```python
from build123d import *

# Parameters (mm, degrees)
F1_DEPTH = 0.15
F2_DEPTH = 1.9
F3_W     = 0.15
F3_H     = 7
F4_DEPTH = 8
F6_DEPTH = 25
F7_R     = 0.5


with BuildPart() as f1:
    # F0 (on Top) → F1 (new body)
    with BuildSketch(Plane.XY):
        with BuildLine():
            Line((96.425, -0.5), (96.425, -3.5))
            Line((96.425, -3.5), (99.425, -3.5))
            Line((99.425, -3.5), (110.2, -3.5))
            Line((110.2, -3.5), (123.975, -3.5))
            Line((123.975, -3.5), (123.975, -0.5))
            Line((123.975, -0.5), (119.375, -0.5))
            ThreePointArc((119.375, -0.5), (119.0921572875, -0.3828427125), (118.975, -0.1))
            Line((118.975, -0.1), (118.975, 0.1))
            ThreePointArc((118.975, 0.1), (119.0921572875, 0.3828427125), (119.375, 0.5))
            Line((119.375, 0.5), (123.975, 0.5))
            Line((123.975, 0.5), (123.975, 3.5))
            Line((123.975, 3.5), (110.2, 3.5))
            Line((110.2, 3.5), (99.425, 3.5))
            Line((99.425, 3.5), (96.425, 3.5))
            Line((96.425, 3.5), (96.425, 0.5))
            Line((96.425, 0.5), (101.025, 0.5))
            ThreePointArc((101.025, 0.5), (101.3078427125, 0.3828427125), (101.425, 0.1))
            Line((101.425, 0.1), (101.425, -0.1))
            ThreePointArc((101.425, -0.1), (101.3078427125, -0.3828427125), (101.025, -0.5))
            Line((101.025, -0.5), (96.425, -0.5))
        make_face()
        with BuildLine():
            Line((13.775, -0.5), (13.775, -3.5))
            Line((13.775, -3.5), (27.55, -3.5))
            Line((27.55, -3.5), (41.325, -3.5))
            Line((41.325, -3.5), (41.325, -0.5))
            Line((41.325, -0.5), (36.725, -0.5))
            ThreePointArc((36.725, -0.5), (36.4421572875, -0.3828427125), (36.325, -0.1))
            Line((36.325, -0.1), (36.325, 0.1))
            ThreePointArc((36.325, 0.1), (36.4421572875, 0.3828427125), (36.725, 0.5))
            Line((36.725, 0.5), (41.325, 0.5))
            Line((41.325, 0.5), (41.325, 3.5))
            Line((41.325, 3.5), (27.55, 3.5))
            Line((27.55, 3.5), (13.775, 3.5))
            Line((13.775, 3.5), (13.775, 0.5))
            Line((13.775, 0.5), (18.375, 0.5))
            ThreePointArc((18.375, 0.5), (18.6578427125, 0.3828427125), (18.775, 0.1))
            Line((18.775, 0.1), (18.775, -0.1))
            ThreePointArc((18.775, -0.1), (18.6578427125, -0.3828427125), (18.375, -0.5))
            Line((18.375, -0.5), (13.775, -0.5))
        make_face()
        with BuildLine():
            Line((41.325, -0.5), (41.325, -3.5))
            Line((41.325, -3.5), (55.1, -3.5))
            Line((55.1, -3.5), (68.875, -3.5))
            Line((68.875, -3.5), (68.875, -0.5))
            Line((68.875, -0.5), (64.275, -0.5))
            ThreePointArc((64.275, -0.5), (63.9921572875, -0.3828427125), (63.875, -0.1))
            Line((63.875, -0.1), (63.875, 0.1))
            ThreePointArc((63.875, 0.1), (63.9921572875, 0.3828427125), (64.275, 0.5))
            Line((64.275, 0.5), (68.875, 0.5))
            Line((68.875, 0.5), (68.875, 3.5))
            Line((68.875, 3.5), (55.1, 3.5))
            Line((55.1, 3.5), (41.325, 3.5))
            Line((41.325, 3.5), (41.325, 0.5))
            Line((41.325, 0.5), (45.925, 0.5))
            ThreePointArc((45.925, 0.5), (46.2078427125, 0.3828427125), (46.325, 0.1))
            Line((46.325, 0.1), (46.325, -0.1))
            ThreePointArc((46.325, -0.1), (46.2078427125, -0.3828427125), (45.925, -0.5))
            Line((45.925, -0.5), (41.325, -0.5))
        make_face()
        with BuildLine():
            Line((68.875, -0.5), (68.875, -3.5))
            Line((68.875, -3.5), (82.65, -3.5))
            Line((82.65, -3.5), (96.425, -3.5))
            Line((96.425, -3.5), (96.425, -0.5))
            Line((96.425, -0.5), (91.825, -0.5))
            ThreePointArc((91.825, -0.5), (91.5421572875, -0.3828427125), (91.425, -0.1))
            Line((91.425, -0.1), (91.425, 0.1))
            ThreePointArc((91.425, 0.1), (91.5421572875, 0.3828427125), (91.825, 0.5))
            Line((91.825, 0.5), (96.425, 0.5))
            Line((96.425, 0.5), (96.425, 3.5))
            Line((96.425, 3.5), (82.65, 3.5))
            Line((82.65, 3.5), (68.875, 3.5))
            Line((68.875, 3.5), (68.875, 0.5))
            Line((68.875, 0.5), (73.475, 0.5))
            ThreePointArc((73.475, 0.5), (73.7578427125, 0.3828427125), (73.875, 0.1))
            Line((73.875, 0.1), (73.875, -0.1))
            ThreePointArc((73.875, -0.1), (73.7578427125, -0.3828427125), (73.475, -0.5))
            Line((73.475, -0.5), (68.875, -0.5))
        make_face()
        with BuildLine():
            Line((0, 3.5), (0, -3.5))
            Line((0, -3.5), (13.775, -3.5))
            Line((13.775, -3.5), (13.775, -0.5))
            Line((13.775, -0.5), (9.175, -0.5))
            ThreePointArc((9.175, -0.5), (8.8921572875, -0.3828427125), (8.775, -0.1))
            Line((8.775, -0.1), (8.775, 0.1))
            ThreePointArc((8.775, 0.1), (8.8921572875, 0.3828427125), (9.175, 0.5))
            Line((9.175, 0.5), (13.775, 0.5))
            Line((13.775, 0.5), (13.775, 3.5))
            Line((13.775, 3.5), (0, 3.5))
        make_face()
        with BuildLine():
            Line((123.975, -0.5), (123.975, -3.5))
            Line((123.975, -3.5), (137.75, -3.5))
            Line((137.75, -3.5), (151.525, -3.5))
            Line((151.525, -3.5), (151.525, -0.5))
            Line((151.525, -0.5), (146.925, -0.5))
            ThreePointArc((146.925, -0.5), (146.6421572875, -0.3828427125), (146.525, -0.1))
            Line((146.525, -0.1), (146.525, 0.1))
            ThreePointArc((146.525, 0.1), (146.6421572875, 0.3828427125), (146.925, 0.5))
            Line((146.925, 0.5), (151.525, 0.5))
            Line((151.525, 0.5), (151.525, 3.5))
            Line((151.525, 3.5), (137.75, 3.5))
            Line((137.75, 3.5), (123.975, 3.5))
            Line((123.975, 3.5), (123.975, 0.5))
            Line((123.975, 0.5), (128.575, 0.5))
            ThreePointArc((128.575, 0.5), (128.8578427125, 0.3828427125), (128.975, 0.1))
            Line((128.975, 0.1), (128.975, -0.1))
            ThreePointArc((128.975, -0.1), (128.8578427125, -0.3828427125), (128.575, -0.5))
            Line((128.575, -0.5), (123.975, -0.5))
        make_face()
        with BuildLine():
            Line((151.525, -0.5), (151.525, -3.5))
            Line((151.525, -3.5), (165.3, -3.5))
            Line((165.3, -3.5), (179.075, -3.5))
            Line((179.075, -3.5), (179.075, -0.5))
            Line((179.075, -0.5), (174.475, -0.5))
            ThreePointArc((174.475, -0.5), (174.1921572875, -0.3828427125), (174.075, -0.1))
            Line((174.075, -0.1), (174.075, 0.1))
            ThreePointArc((174.075, 0.1), (174.1921572875, 0.3828427125), (174.475, 0.5))
            Line((174.475, 0.5), (179.075, 0.5))
            Line((179.075, 0.5), (179.075, 3.5))
            Line((179.075, 3.5), (165.3, 3.5))
            Line((165.3, 3.5), (151.525, 3.5))
            Line((151.525, 3.5), (151.525, 0.5))
            Line((151.525, 0.5), (156.125, 0.5))
            ThreePointArc((156.125, 0.5), (156.4078427125, 0.3828427125), (156.525, 0.1))
            Line((156.525, 0.1), (156.525, -0.1))
            ThreePointArc((156.525, -0.1), (156.4078427125, -0.3828427125), (156.125, -0.5))
            Line((156.125, -0.5), (151.525, -0.5))
        make_face()
        with BuildLine():
            Line((179.075, -0.5), (179.075, -3.5))
            Line((179.075, -3.5), (192.85, -3.5))
            Line((192.85, -3.5), (206.625, -3.5))
            Line((206.625, -3.5), (206.625, -0.5))
            Line((206.625, -0.5), (202.025, -0.5))
            ThreePointArc((202.025, -0.5), (201.7421572875, -0.3828427125), (201.625, -0.1))
            Line((201.625, -0.1), (201.625, 0.1))
            ThreePointArc((201.625, 0.1), (201.7421572875, 0.3828427125), (202.025, 0.5))
            Line((202.025, 0.5), (206.625, 0.5))
            Line((206.625, 0.5), (206.625, 3.5))
            Line((206.625, 3.5), (192.85, 3.5))
            Line((192.85, 3.5), (179.075, 3.5))
            Line((179.075, 3.5), (179.075, 0.5))
            Line((179.075, 0.5), (183.675, 0.5))
            ThreePointArc((183.675, 0.5), (183.9578427125, 0.3828427125), (184.075, 0.1))
            Line((184.075, 0.1), (184.075, -0.1))
            ThreePointArc((184.075, -0.1), (183.9578427125, -0.3828427125), (183.675, -0.5))
            Line((183.675, -0.5), (179.075, -0.5))
        make_face()
    extrude(amount=F1_DEPTH)

    # F2 (add): a face of the model
    f2_faces = [f1.faces().sort_by_distance(p)[0] for p in [
        (0, 0, 0.075),
    ]]
    extrude(f2_faces, amount=F2_DEPTH)

    # F3 (on face) → F4 (join)
    with BuildSketch(Plane(origin=(0, 0, 0), x_dir=(1, 0, 0), z_dir=(0, 0, -1))):
        with Locations((-1.825, 0)):
            Rectangle(F3_W, F3_H)
    extrude(amount=F4_DEPTH)

    # F5 (on face) → F6 (cut)
    with BuildSketch(Plane(origin=(-1.9, 0, 0), x_dir=(0, -1, 0), z_dir=(-1, 0, 0))):
        with BuildLine():
            ThreePointArc((0.5, -7.1), (0.3828427125, -6.8171572875), (0.1, -6.7))
            Line((0.1, -6.7), (-0.1, -6.7))
            ThreePointArc((-0.1, -6.7), (-0.3828427125, -6.8171572875), (-0.5, -7.1))
            Line((-0.5, -7.1), (-0.5, -8))
            Line((-0.5, -8), (0.5, -8))
            Line((0.5, -8), (0.5, -7.1))
        make_face()
    extrude(amount=-F6_DEPTH, mode=Mode.SUBTRACT)

    # F7
    f7_edges = [f1.edges().sort_by_distance(p)[0] for p in [
        (-1.9, 0, 0.15),
        (-1.75, 0, 0),
    ]]
    fillet(f7_edges, radius=F7_R)


solid = f1.part
```
Geometry check sheet. Reference: the model listing, model coordinates, mm. Give positions to 0.01 mm unless a question says otherwise; leave off trailing zeros. Write each loop counter-clockwise with the first axis right and the second up, starting at its lowest first coordinate (ties: lowest second). Pieces come first, ordered by that corner, then holes. Notation, with made-up numbers: (79.25, 57.5) -> (93.25, 57.5) arc R18 cw to (93.25, 87.5) -> close; hole circle Ø7 at (-3, 67.5). An arc over 180 degrees is marked (long way). Use one line per item in the form item = value.
Item 1: Sectioned sample at A-A on y = 2. Enter the section's corners in (x, z) (3 decimals), plus the area to 3 significant figures.
Results list:
outline = (-1.9, -8) -> (-1.75, -8) -> (-1.75, -0.5) arc R0.5 cw to (-1.25, 0) -> (206.625, 0) -> (206.625, 0.15) -> (-1.4, 0.15) arc R0.5 ccw to (-1.9, -0.35) -> close
area = 32.5 mm2
Item 2: Scan lines: line 1 (Z direction, x = 183, y = 2.75); line 2 (X direction, y = 3.25, z = -0.25). Record each from-to range of solid material in increasing order.
Results list:
line_1 = 0 to 0.15
line_2 = -1.89 to -1.68
Item 3: Depth check by flat-ended pin: pin 1 Ø3 at (x, y) = (86.5, -1.5) entering from -Z; pin 2 Ø3 at (x, z) = (29.5, -2.5) entering from -Y. Enter the tip coordinate at first touch or a pass-through.
Results list:
pin_1 = 0
pin_2 = through
Item 4: Sectioned sample at C-C on z = -4.5. Enter the section's corners in (x, y), plus the area to 3 significant figures.
Results list:
outline = (-1.9, -3.5) -> (-1.75, -3.5) -> (-1.75, 3.5) -> (-1.9, 3.5) -> close
area = 1.05 mm2
Item 5: Sectioned sample at B-B on x = 30. Enter the section's corners in (y, z), plus the area to 3 significant figures.
Results list:
outline = (-3.5, 0) -> (3.5, 0) -> (3.5, 0.15) -> (-3.5, 0.15) -> close
area = 1.05 mm2
